from build123d import *

# Parameters (mm, degrees)
Y_KSEKLIK_EKSTR_ZYON2_DEPTH = 40


with BuildPart() as part:
    # Çizim1 → Yükseklik-Ekstrüzyon2 (new body)
    with BuildSketch(Plane.XY):
        with BuildLine():
            ThreePointArc((-12.75, -4.6), (-12.896446609, -4.246446609), (-13.25, -4.1))
            Line((-13.25, -4.1), (-14.35, -4.1))
            ThreePointArc((-14.35, -4.1), (-14.456066017, -4.143933983), (-14.5, -4.25))
            Line((-14.5, -4.25), (-14.5, -4.7))
            ThreePointArc((-14.5, -4.7), (-14.543933983, -4.806066017), (-14.65, -4.85))
            Line((-14.65, -4.85), (-14.85, -4.85))
            ThreePointArc((-14.85, -4.85), (-14.956066017, -4.893933983), (-15, -5))
            Line((-15, -5), (-15, -13.5))
            ThreePointArc((-15, -13.5), (-14.560660172, -14.560660172), (-13.5, -15))
            Line((-13.5, -15), (-5, -15))
            ThreePointArc((-5, -15), (-4.893933983, -14.956066017), (-4.85, -14.85))
            Line((-4.85, -14.85), (-4.85, -14.65))
            ThreePointArc((-4.85, -14.65), (-4.806066017, -14.543933983), (-4.7, -14.5))
            Line((-4.7, -14.5), (-4.25, -14.5))
            ThreePointArc((-4.25, -14.5), (-4.143933983, -14.456066017), (-4.1, -14.35))
            Line((-4.1, -14.35), (-4.1, -13.25))
            ThreePointArc((-4.1, -13.25), (-4.246446609, -12.896446609), (-4.6, -12.75))
            Line((-4.6, -12.75), (-8.25, -12.75))
            ThreePointArc((-8.25, -12.75), (-8.603553391, -12.603553391), (-8.75, -12.25))
            Line((-8.75, -12.25), (-8.75, -10.548097039))
            ThreePointArc((-8.75, -10.548097039), (-8.711939766, -10.356755323), (-8.603553391, -10.194543648))
            Line((-8.603553391, -10.194543648), (-5.665324285, -7.256314543))
            ThreePointArc((-5.665324285, -7.256314543), (-3.584805828, -6.008237883), (-1.161703843, -5.88646279))
            ThreePointArc((-1.161703843, -5.88646279), (0.121501595, -5.998769654), (1.399107062, -5.834595053))
            ThreePointArc((1.399107062, -5.834595053), (3.922877314, -5.884663497), (6.100563519, -7.161223691))
            Line((6.100563519, -7.161223691), (8.060660172, -9.121320344))
            ThreePointArc((8.060660172, -9.121320344), (8.385819299, -9.607955367), (8.5, -10.181980515))
            Line((8.5, -10.181980515), (8.5, -12.25))
            ThreePointArc((8.5, -12.25), (8.353553391, -12.603553391), (8, -12.75))
            Line((8, -12.75), (4.6, -12.75))
            ThreePointArc((4.6, -12.75), (4.246446609, -12.896446609), (4.1, -13.25))
            Line((4.1, -13.25), (4.1, -14.35))
            ThreePointArc((4.1, -14.35), (4.143933983, -14.456066017), (4.25, -14.5))
            Line((4.25, -14.5), (4.7, -14.5))
            ThreePointArc((4.7, -14.5), (4.806066017, -14.543933983), (4.85, -14.65))
            Line((4.85, -14.65), (4.85, -14.85))
            ThreePointArc((4.85, -14.85), (4.893933983, -14.956066017), (5, -15))
            Line((5, -15), (13.5, -15))
            ThreePointArc((13.5, -15), (14.560660172, -14.560660172), (15, -13.5))
            Line((15, -13.5), (15, -10.020449132))
            ThreePointArc((15, -10.020449132), (7.671680118, 7.671680118), (-10.020449132, 15))
            Line((-10.020449132, 15), (-13.5, 15))
            ThreePointArc((-13.5, 15), (-14.560660172, 14.560660172), (-15, 13.5))
            Line((-15, 13.5), (-15, 5))
            ThreePointArc((-15, 5), (-14.956066017, 4.893933983), (-14.85, 4.85))
            Line((-14.85, 4.85), (-14.65, 4.85))
            ThreePointArc((-14.65, 4.85), (-14.543933983, 4.806066017), (-14.5, 4.7))
            Line((-14.5, 4.7), (-14.5, 4.25))
            ThreePointArc((-14.5, 4.25), (-14.456066017, 4.143933983), (-14.35, 4.1))
            Line((-14.35, 4.1), (-13.25, 4.1))
            ThreePointArc((-13.25, 4.1), (-12.896446609, 4.246446609), (-12.75, 4.6))
            Line((-12.75, 4.6), (-12.75, 8))
            ThreePointArc((-12.75, 8), (-12.603553391, 8.353553391), (-12.25, 8.5))
            Line((-12.25, 8.5), (-10.181980515, 8.5))
            ThreePointArc((-10.181980515, 8.5), (-9.607955367, 8.385819299), (-9.121320344, 8.060660172))
            Line((-9.121320344, 8.060660172), (-7.161223691, 6.100563519))
            ThreePointArc((-7.161223691, 6.100563519), (-5.884663497, 3.922877314), (-5.834595053, 1.399107062))
            ThreePointArc((-5.834595053, 1.399107062), (-5.998769654, 0.121501595), (-5.88646279, -1.161703843))
            ThreePointArc((-5.88646279, -1.161703843), (-6.008237883, -3.584805828), (-7.256314543, -5.665324285))
            Line((-7.256314543, -5.665324285), (-10.103553391, -8.512563133))
            ThreePointArc((-10.103553391, -8.512563133), (-10.265765065, -8.620949509), (-10.457106781, -8.659009742))
            Line((-10.457106781, -8.659009742), (-12.25, -8.659009742))
            ThreePointArc((-12.25, -8.659009742), (-12.603553391, -8.512563133), (-12.75, -8.159009742))
            Line((-12.75, -8.159009742), (-12.75, -4.6))
        make_face()
        with BuildLine():
            ThreePointArc((2.587626892, 5.413334191), (0.660394354, 5.963545866), (-1.340526419, 5.848332149))
            ThreePointArc((-1.340526419, 5.848332149), (-4.339403848, 5.930394105), (-6.923693524, 7.45402361))
            Line((-6.923693524, 7.45402361), (-9.030330086, 9.560660172))
            ThreePointArc((-9.030330086, 9.560660172), (-9.516965109, 9.885819299), (-10.090990258, 10))
            Line((-10.090990258, 10), (-13, 10))
            ThreePointArc((-13, 10), (-13.353553391, 10.146446609), (-13.5, 10.5))
            Line((-13.5, 10.5), (-13.5, 13))
            ThreePointArc((-13.5, 13), (-13.353553391, 13.353553391), (-13, 13.5))
            Line((-13, 13.5), (-10.020449132, 13.5))
            ThreePointArc((-10.020449132, 13.5), (-2.058398163, 11.971373122), (4.771466284, 7.602859941))
            ThreePointArc((4.771466284, 7.602859941), (5.02983183, 7.200254947), (5.071628638, 6.723708451))
            ThreePointArc((5.071628638, 6.723708451), (4.158873557, 5.444388853), (2.587626892, 5.413334191))
        make_face(mode=Mode.SUBTRACT)
        with BuildLine():
            ThreePointArc((5.848332149, -1.340526419), (5.963545866, 0.660394354), (5.413334191, 2.587626892))
            ThreePointArc((5.413334191, 2.587626892), (5.444388853, 4.158873557), (6.723708451, 5.071628638))
            ThreePointArc((6.723708451, 5.071628638), (7.200254947, 5.02983183), (7.602859941, 4.771466284))
            ThreePointArc((7.602859941, 4.771466284), (11.971373122, -2.058398163), (13.5, -10.020449132))
            Line((13.5, -10.020449132), (13.5, -13))
            ThreePointArc((13.5, -13), (13.353553391, -13.353553391), (13, -13.5))
            Line((13, -13.5), (10.5, -13.5))
            ThreePointArc((10.5, -13.5), (10.146446609, -13.353553391), (10, -13))
            Line((10, -13), (10, -10.090990258))
            ThreePointArc((10, -10.090990258), (9.885819299, -9.516965109), (9.560660172, -9.030330086))
            Line((9.560660172, -9.030330086), (7.45402361, -6.923693524))
            ThreePointArc((7.45402361, -6.923693524), (5.930394105, -4.339403848), (5.848332149, -1.340526419))
        make_face(mode=Mode.SUBTRACT)
        with BuildLine():
            Line((-13.25, -12.75), (-13.25, -10.75))
            ThreePointArc((-13.25, -10.75), (-13.103553391, -10.396446609), (-12.75, -10.25))
            Line((-12.75, -10.25), (-10.75, -10.25))
            ThreePointArc((-10.75, -10.25), (-10.396446609, -10.396446609), (-10.25, -10.75))
            Line((-10.25, -10.75), (-10.25, -12.75))
            ThreePointArc((-10.25, -12.75), (-10.396446609, -13.103553391), (-10.75, -13.25))
            Line((-10.75, -13.25), (-12.75, -13.25))
            ThreePointArc((-12.75, -13.25), (-13.103553391, -13.103553391), (-13.25, -12.75))
        make_face(mode=Mode.SUBTRACT)
        with BuildLine():
            ThreePointArc((2.545584412, 3.606244584), (3.075914498, 3.825914498), (3.606244584, 3.606244584))
            ThreePointArc((3.606244584, 3.606244584), (3.825914498, 3.075914498), (3.606244584, 2.545584412))
            Line((3.606244584, 2.545584412), (2.947715037, 1.887054865))
            ThreePointArc((2.947715037, 1.887054865), (3.5, 0), (2.947715037, -1.887054865))
            Line((2.947715037, -1.887054865), (3.606244584, -2.545584412))
            ThreePointArc((3.606244584, -2.545584412), (3.606244584, -3.606244584), (2.545584412, -3.606244584))
            Line((2.545584412, -3.606244584), (1.887054865, -2.947715037))
            ThreePointArc((1.887054865, -2.947715037), (0, -3.5), (-1.887054865, -2.947715037))
            Line((-1.887054865, -2.947715037), (-2.545584412, -3.606244584))
            ThreePointArc((-2.545584412, -3.606244584), (-3.606244584, -3.606244584), (-3.606244584, -2.545584412))
            Line((-3.606244584, -2.545584412), (-2.947715037, -1.887054865))
            ThreePointArc((-2.947715037, -1.887054865), (-3.5, 0), (-2.947715037, 1.887054865))
            Line((-2.947715037, 1.887054865), (-3.606244584, 2.545584412))
            ThreePointArc((-3.606244584, 2.545584412), (-3.606244584, 3.606244584), (-2.545584412, 3.606244584))
            Line((-2.545584412, 3.606244584), (-1.887054865, 2.947715037))
            ThreePointArc((-1.887054865, 2.947715037), (0, 3.5), (1.887054865, 2.947715037))
            Line((1.887054865, 2.947715037), (2.545584412, 3.606244584))
        make_face(mode=Mode.SUBTRACT)
    extrude(amount=-Y_KSEKLIK_EKSTR_ZYON2_DEPTH)


solid = part.part
Verification items for the finished model (mm, model axes). A direction names the side the tool comes from. Coordinates: 2 decimals unless noted, no trailing zeros. Write each loop counter-clockwise with the first axis right and the second up, starting at its lowest first coordinate (ties: lowest second). Pieces come first, ordered by that corner, then holes. Notation, with made-up numbers: (54, 86) - (69, 86) arc R6 cw to (69, 97) - close; hole circle Ø9 at (20, 46.25). An arc over 180 degrees is marked (long way). Answer as a JSON object with one key per item and string values.
(1) Tool access check on faces 4 (the flat face through (-9, -15, -20)), 5 (the flat face through (-14, 4.1, -20)), 6 (the flat face through (-12.75, 6, -20)). Record the directions out of +Z, -Z, +X, -X, +Y, -Y that give a thin tool (end or side, any length) a straight path to the whole face; none if there is none.
Report:
{"face 4": "+Z, -Z, +X, -X, -Y", "face 5": "+Z, -Z, -X", "face 6": "+Z, -Z"}
(2) Gauge pin test, flat ends, axial feed: pin 1 Ø4 at (y, z) = (0.5, -13.5) entering from +X; pin 2 Ø2 at (x, z) = (8.5, -22) entering from +Y; pin 3 Ø5 at (x, z) = (4.5, -33.5) entering from +Y. Record the tip position at first contact, or that the pin passes through.
Report:
{"pin 1": "x = 13.5", "pin 2": "y = 7.84", "pin 3": "y = 11.92"}
(3) Cross-section at A-A on y = -11.75. Record the cut outline in (x, z), plus the area to 3 significant figures.
Report:
{"outline": "(-15, -40) - (-13.25, -40) - (-13.25, 0) - (-15, 0) - close; (-10.25, -40) - (-8.75, -40) - (-8.75, 0) - (-10.25, 0) - close; (8.5, -40) - (10, -40) - (10, 0) - (8.5, 0) - close; (13.5, -40) - (15, -40) - (15, 0) - (13.5, 0) - close", "area": "250 mm^2"}
(4) Cross-section at C-C on x = 11.5. Record the cut outline in (y, z), plus the area to 3 significant figures.
Report:
{"outline": "(-15, -40) - (-13.5, -40) - (-13.5, 0) - (-15, 0) - close; (-0.97, -40) - (2.74, -40) - (2.74, 0) - (-0.97, 0) - close", "area": "208 mm^2"}
(5) Mould release check, pull along Y, two halves, no side actions. Record for faces 1 (the flat face through (9, -15, -20)), 2 (the cylindrical face through (3.5, 0, -19.7)), 3 (the flat face through (-4.1, -14, -20)): pulls with the +Y half, pulls with the -Y half, needs draft (parallel to the pull), parting line crosses it, or undercut.
Report:
{"face 1": "pulls with the -Y half", "face 2": "undercut", "face 3": "needs draft"}
(6) Cross-section at D-D on z = -10. Give the number of separate pieces and of enclosed holes in the cut face, plus the area to 3 significant figures.
Report:
{"separate pieces": "1", "enclosed holes": "4", "area": "291 mm^2"}
(7) Thickness scan on line 1 along X through (y, z) = (-11, -2); line 2 along Y through (x, z) = (-5, -14.5); line 3 along Y through (x, z) = (7.75, -23). Record the ranges inside material, lowest first.
Report:
{"line 1": "-15 to -13.25, -10.25 to -8.75, 8.5 to 10, 13.5 to 15", "line 2": "-15 to -12.75, -6.7 to 6.16, 12.91 to 14.49", "line 3": "-15 to -12.75, -8.81 to -7.22, 4.61 to 7.59"}
(8) Cross-section at B-B on y = 0.25. Record the cut outline in (x, z).
Report:
{"outline": "(-5.99, -40) - (-3.49, -40) - (-3.49, 0) - (-5.99, 0) - close; (3.49, -40) - (5.99, -40) - (5.99, 0) - (3.49, 0) - close; (10.89, -40) - (12.79, -40) - (12.79, 0) - (10.89, 0) - close"}
